Check sheet for the modelled part. Datum: model origin and axes. Units: mm. Face numbers are marked on the shaded views. A direction names the side the tool comes from. Coordinates: 2 decimals unless noted, no trailing zeros. Write each loop counter-clockwise with the first axis right and the second up, starting at its lowest first coordinate (ties: lowest second). Pieces come first, ordered by that corner, then holes. Notation, with made-up numbers: (-1, 14.5) - (44, 14.5) arc R23 cw to (44, 40.5) - close; hole circle Ø2 at (73.5, -30.75). An arc over 180 degrees is marked (long way). Write each question's results on one line, items separated by ' | '.
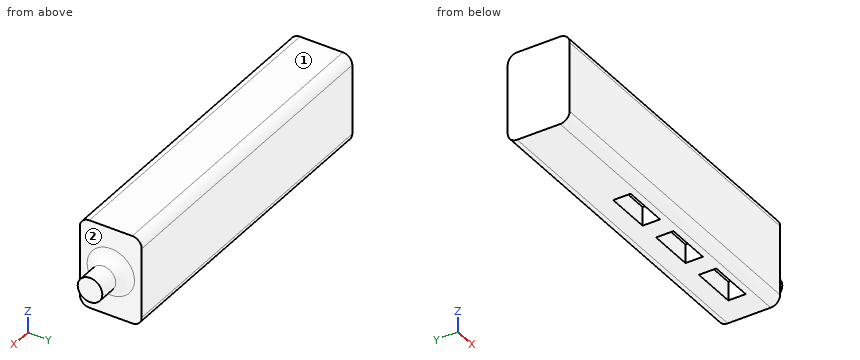
from build123d import *

# Parameters (mm, degrees)
BOSS_EXTRUDE1_DEPTH = 43
SKETCH2_R           = 3.25
BOSS_EXTRUDE2_DEPTH = 8.5
FILLET1_R           = 3
SKETCH3_W           = 12
SKETCH3_H           = 4.6
CUT_EXTRUDE1_DEPTH  = 5


with BuildPart() as part:
    # Sketch1 → Boss-Extrude1 (new, symmetric)
    with BuildSketch(Plane(origin=(0, 0, 0), x_dir=(0, 0, -1), z_dir=(1, 0, 0))):
        with BuildLine():
            Line((-9.25, -8.175), (9.25, -8.175))
            ThreePointArc((9.25, -8.175), (11.017766953, -7.442766953), (11.75, -5.675))
            Line((11.75, -5.675), (11.75, 5.675))
            ThreePointArc((11.75, 5.675), (11.017766953, 7.442766953), (9.25, 8.175))
            Line((9.25, 8.175), (-9.25, 8.175))
            ThreePointArc((-9.25, 8.175), (-11.017766953, 7.442766953), (-11.75, 5.675))
            Line((-11.75, 5.675), (-11.75, -5.675))
            ThreePointArc((-11.75, -5.675), (-11.017766953, -7.442766953), (-9.25, -8.175))
        make_face()
    extrude(amount=BOSS_EXTRUDE1_DEPTH, both=True)

    # Sketch2 → Boss-Extrude2 (add)
    with BuildSketch(Plane(origin=(43, 0, 0), x_dir=(0, 0, -1), z_dir=(1, 0, 0))):
        with Locations(Location((0, 0, 0), (0, 0, 180))):
            Circle(SKETCH2_R)
    extrude(amount=BOSS_EXTRUDE2_DEPTH)

    # Fillet1
    fillet1_edges = [part.edges().sort_by_distance(p)[0] for p in [
        (43, 0, -3.25),
    ]]
    fillet(fillet1_edges, radius=FILLET1_R)

    # Sketch3 → Cut-Extrude1 (cut)
    with BuildSketch(Plane(origin=(0, 0, -11.75), x_dir=(-1, 0, 0), z_dir=(0, 0, -1))):
        with Locations((5.5, -1.625)):
            Rectangle(SKETCH3_W, SKETCH3_H)
        with Locations((-12, -1.625)):
            Rectangle(SKETCH3_W, SKETCH3_H)
        with Locations((-29.5, -1.625)):
            Rectangle(SKETCH3_W, SKETCH3_H)
    extrude(amount=-CUT_EXTRUDE1_DEPTH, mode=Mode.SUBTRACT)


solid = part.part
1. Sectioned sample at B-B (z = 0). Record the cut outline in (x, y) (3 decimals), then the cut area to 3 significant figures.
Values follow:
outline: (-43, -8.175) - (43, -8.175) - (43, -6.25) arc R3 cw to (46, -3.25) - (51.5, -3.25) - (51.5, 3.25) - (46, 3.25) arc R3 cw to (43, 6.25) - (43, 8.175) - (-43, 8.175) - close | area: 1,470 mm^2
2. Material ranges on L1, parallel to X at y = -2, z = -7.5; L2, parallel to X at y = 5.5, z = 10.75; L3, parallel to Z at x = 38, y = 5.75, recorded low to high. Write a range as [from, to].
Values follow:
L1: x = [-43, -11.5], [0.5, 6], [18, 23.5], [35.5, 43] | L2: x = [-43, 43] | L3: z = [-11.75, 11.75]
3. Sectioned sample at A-A (x = -10.5). Record the cut outline in (y, z) (3 decimals).
Values follow:
outline: (-8.175, -9.25) arc R2.5 ccw to (-5.675, -11.75) - (-3.925, -11.75) - (-3.925, -6.75) - (0.675, -6.75) - (0.675, -11.75) - (5.675, -11.75) arc R2.5 ccw to (8.175, -9.25) - (8.175, 9.25) arc R2.5 ccw to (5.675, 11.75) - (-5.675, 11.75) arc R2.5 ccw to (-8.175, 9.25) - close
4. Access from +Z, -Z, +X, -X, +Y, -Y to the whole of each face (thin tool, end or side, straight path). Record for the marked faces 1 and 2.
Values follow:
face 1: +Z, +X, -X, +Y, -Y | face 2: +X
5. Go/stop test with flat-tipped pins: pin 1 (8 mm diameter, centred on y = 2, z = 4, fed in from +X); pin 2 (5 mm diameter, centred on y = -0.5, z = -8, fed in from +X); pin 3 (3.5 mm diameter, centred on x = -7.5, y = -2, fed in from -Z). Record where each tip stops, or that it passes through.
Values follow:
pin 1: stops at x = 51.5 | pin 2: stops at x = 43.09 | pin 3: stops at z = -6.75
6. Sectioned sample at C-C (z = 7.75). Record the cut outline in (x, y) (3 decimals).
Values follow:
outline: (-43, -8.175) - (43, -8.175) - (43, 8.175) - (-43, 8.175) - close
